from build123d import *

# Parameters (mm, degrees)
SKETCH1_W            = 30
SKETCH1_H            = 30
SKETCH1_W_2          = 12
SKETCH1_H_2          = 26
BOSS_EXTRUDE2_DEPTH  = 100
SKETCH3_W            = 7
SKETCH3_H            = 26
CUT_EXTRUDE2_DEPTH   = 70
FILLET1_R            = 15
SKETCH5_R            = 4
CUT_EXTRUDE3_DEPTH   = 50
SKETCH6_R            = 11.3
CUT_EXTRUDE4_DEPTH   = 7.4
CUT_EXTRUDE5_START   = -7.4
SKETCH7_R            = 11.3
CUT_EXTRUDE5_DEPTH   = 7.4
M3_CLEARANCE_HOLE1_D = 3.6


with BuildPart() as part:
    # Sketch1 → Boss-Extrude2 (new body)
    with BuildSketch(Plane(origin=(0, 0, 0), x_dir=(1, 0, 0), z_dir=(0, 1, 0))):
        Rectangle(SKETCH1_W, SKETCH1_H)
        Rectangle(SKETCH1_W_2, SKETCH1_H_2, mode=Mode.SUBTRACT)
    extrude(amount=BOSS_EXTRUDE2_DEPTH)

    # Sketch3 → Cut-Extrude2 (cut)
    with BuildSketch(Plane(origin=(0, 100, 0), x_dir=(1, 0, 0), z_dir=(0, 1, 0))):
        with Locations((-9.5, 0)):
            Rectangle(SKETCH3_W, SKETCH3_H)
        with Locations((9.5, 0)):
            Rectangle(SKETCH3_W, SKETCH3_H)
    extrude(amount=-CUT_EXTRUDE2_DEPTH, mode=Mode.SUBTRACT)

    # Fillet1
    # the kernel refuses this fillet: 15 mm, written as the material it takes off along each edge
    with BuildSketch(Plane(origin=(52.5, 0, -15), x_dir=(0, 1, 0), z_dir=(-1, 0, 0)), Plane(origin=(-52.5, 0, 15), x_dir=(0, 1, 0), z_dir=(1, 0, 0))) as fillet1_piece_1:
        with BuildLine():
            CenterArc((FILLET1_R, -FILLET1_R), FILLET1_R, 90, 90)
            Line((0, -FILLET1_R), (0, 0))
            Line((0, 0), (FILLET1_R, 0))
        make_face()
    extrude(amount=105, mode=Mode.SUBTRACT)

    # Sketch5 → Cut-Extrude3 (cut)
    with BuildSketch(Plane(origin=(15, 0, 0), x_dir=(0, 0, -1), z_dir=(1, 0, 0))):
        with Locations((0, 15)):
            Circle(SKETCH5_R)
    extrude(amount=-CUT_EXTRUDE3_DEPTH, mode=Mode.SUBTRACT)

    # Sketch6 → Cut-Extrude4 (cut)
    with BuildSketch(Plane(origin=(15, 0, 0), x_dir=(0, 0, -1), z_dir=(1, 0, 0))):
        with Locations((0, 15)):
            Circle(SKETCH6_R)
    extrude(amount=-CUT_EXTRUDE4_DEPTH, mode=Mode.SUBTRACT)

    # Sketch7 → Cut-Extrude5 (cut)
    with BuildSketch(Plane.ZY.offset(15).offset(CUT_EXTRUDE5_START)):
        with Locations(Location((0, 15, 0), (0, 0, 180))):
            Circle(SKETCH7_R)
    extrude(amount=CUT_EXTRUDE5_DEPTH, mode=Mode.SUBTRACT)

    # M3 Clearance Hole1 (through all)
    with Locations(Plane(origin=(15, 0, 0), x_dir=(0, 0, -1), z_dir=(1, 0, 0))):
        with Locations((-10, 95), (-10, 75), (10, 75), (10, 95)):
            Hole(M3_CLEARANCE_HOLE1_D / 2)


solid = part.part
Input: part model. Units: mm. Frame: model coordinates. A direction names the side the tool comes from. Give positions to 0.01 mm unless a question says otherwise; leave off trailing zeros. Write each loop counter-clockwise with the first axis right and the second up, starting at its lowest first coordinate (ties: lowest second). Pieces come first, ordered by that corner, then holes.
Q1. Material intervals for probe 1 along Z at (x, y) = (-14, 95); probe 2 along X at (y, z) = (63, 1), sorted ascending.
Q2. Section A-A, the plane y = 75. Output: boundary loops of the cut face in (x, z), plus the area to 3 significant figures.
Q3. Set-up query: faces 3 (the face through (11.4, 26.2, 1.5)), 4 (the face through (0, 53, -13)), 5 (the face through (-6, 18, 3)). Return all of +Z, -Z, +X, -X, +Y, -Y with unobstructed straight access to the full face (end or side cutting, diameter ignored); none if empty.
Q4. First-contact query: P1, Ø1, axis at x = -4, z = 8.5, coming from the +Y side; P2, Ø7.5, axis at x = 8.5, z = 4.5, coming from the +Y side. Flat tips, straight axial feed; report the tip coordinate or a pass-through.
Q5. Section C-C, the plane y = 55. Output: boundary loops of the cut face in (x, z), plus the area to 3 significant figures.
Q6. Section B-B, the plane x = -1.5. Output: boundary loops of the cut face in (y, z).
Q7. Section D-D, the plane z = -1.75. Output: boundary loops of the cut face in (x, y).
Q8. Pull-direction query (Y, two-part tool) for faces 1 (the face through (13, 65, 0)), 2 (the face through (7.6, 10, 0)); classes: pulls with the +Y half, pulls with the -Y half, needs draft (parallel to the pull), parting line crosses it, or undercut.
Filled in:
1. probe 1: z = -15 to -11.8, -8.2 to 8.2, 11.8 to 15
1. probe 2: x = -15 to -13, 13 to 15
2. outline: (-15, -15) - (15, -15) - (15, -11.8) - (13, -11.8) - (13, -13) - (-13, -13) - (-13, -11.8) - (-15, -11.8) - close; (-15, -8.2) - (-13, -8.2) - (-13, 8.2) - (-15, 8.2) - close; (-15, 11.8) - (-13, 11.8) - (-13, 13) - (13, 13) - (13, 11.8) - (15, 11.8) - (15, 15) - (-15, 15) - close; (13, -8.2) - (15, -8.2) - (15, 8.2) - (13, 8.2) - close
2. area: 195 mm2
3. face 3: +X
3. face 4: +Y
3. face 5: +Y, -Y
4. P1: passes through
4. P2: stops at y = 30
5. outline: (-15, -15) - (15, -15) - (15, 15) - (-15, 15) - close; hole (-13, -13) - (13, -13) - (13, 13) - (-13, 13) - close
5. area: 224 mm2
6. outline: (7.52, -13) arc R15 ccw to (15, -15) - (100, -15) - (100, -13) - close; (7.52, 13) - (100, 13) - (100, 15) - (15, 15) arc R15 ccw to start
7. outline: (-15, 0.1) - (-6, 0.1) - (-6, 11.4) - (-7.6, 11.4) - (-7.6, 3.84) - (-15, 3.84) - close; (-15, 26.16) - (-7.6, 26.16) - (-7.6, 18.6) - (-6, 18.6) - (-6, 30) - (-13, 30) - (-13, 100) - (-15, 100) - close; (6, 0.1) - (15, 0.1) - (15, 3.84) - (7.6, 3.84) - (7.6, 11.4) - (6, 11.4) - close; (6, 18.6) - (7.6, 18.6) - (7.6, 26.16) - (15, 26.16) - (15, 100) - (13, 100) - (13, 30) - (6, 30) - close
8. face 1: needs draft
8. face 2: undercut
